Can you work these out from the model? Positions are in its coordinate system, mm. Round coordinates to 2 decimals unless told otherwise and drop trailing zeros. Write each loop counter-clockwise with the first axis right and the second up, starting at its lowest first coordinate (ties: lowest second). Pieces come first, ordered by that corner, then holes. Notation, with made-up numbers: M -1.5,-11.75 L 43.5,-11.75 A15 cw 43.5,9.25 Z; hole C 62.25,42 d5. An arc over 180 degrees is marked long. Answer as a JSON object with one key per item and string values. Group by question number.
1) Suppose I cut it at C-C, the plane z = -49.5. Write out the boundary of the cut face in (x, y).
2) Please list where these lines run through material, in increasing order: L1, parallel to Y at x = 0.65, z = -45; L2, parallel to Z at x = 0.2, y = -82; L3, parallel to Y at x = 0.6, z = -64. Write a range as [from, to].
3) Suppose I cut it at B-B, the plane y = -74. Write out the boundary of the cut face in (x, z).
4) Suppose I cut it at A-A, the plane x = 0.55. Write out the boundary of the cut face in (y, z), and give its area (3 significant figures).
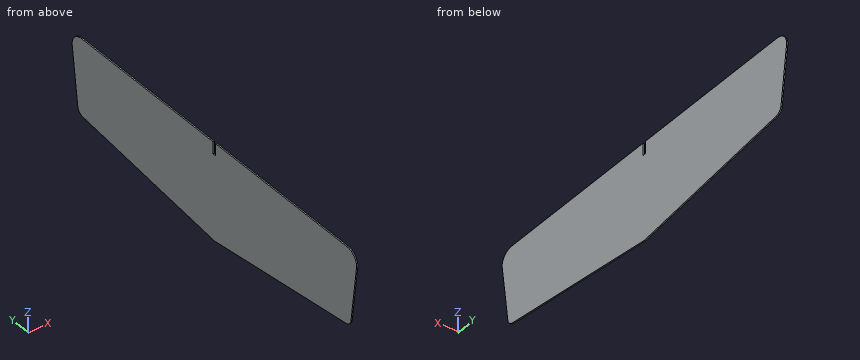
from build123d import *

# Parameters (mm, degrees)
F1_DEPTH = 1


# Not quite as in the source:
# - ends of sketch curves that miss each other by under 0.0002 mm in the source are joined


with BuildPart() as f1:
    # F0 (on Right) → F1 (new body)
    with BuildSketch(Plane.YZ):
        with BuildLine():
            Line((-17.710118, -7.110515), (-155.042295, -7.110515))
            ThreePointArc((-155.042295, -7.110515), (-162.539076635, -10.4924892282), (-164.9650738133, -18.3508619767))
            Line((-164.9650738133, -18.3508619767), (-159.139913, -64.952155))
            ThreePointArc((-159.139913, -64.952155), (-157.4251457547, -68.4543233257), (-153.91996093, -70.1629154318))
            Line((-153.91996093, -70.1629154318), (-16.370118, -87.110515))
            Line((-16.370118, -87.110515), (121.179726, -70.162916))
            ThreePointArc((121.179726, -70.162916), (124.6849107108, -68.4543233695), (126.3996771834, -64.9521550229))
            Line((126.3996771834, -64.9521550229), (132.224839, -18.350862))
            ThreePointArc((132.224839, -18.350862), (129.798841635, -10.4924892282), (122.30206, -7.110515))
            Line((122.30206, -7.110515), (-15.030118, -7.110515))
            Line((-15.030118, -7.110515), (-15.030118, -17.110515))
            Line((-15.030118, -17.110515), (-17.710118, -17.110515))
            Line((-17.710118, -17.110515), (-17.710118, -7.110515))
        make_face()
    extrude(amount=F1_DEPTH)


solid = f1.part
Results:
{
 "1": {"outline": "M 0,-161.07 L 1,-161.07 L 1,128.33 L 0,128.33 Z"},
 "2": {"L1": "[-161.63, 128.89]", "L2": "[-79.02, -7.11]", "L3": "[-159.26, 126.52]"},
 "3": {"outline": "M 0,-80.01 L 1,-80.01 L 1,-7.11 L 0,-7.11 Z"},
 "4": {"outline": "M -164.97,-18.35 L -159.14,-64.95 A6 ccw -153.92,-70.16 L -16.37,-87.11 L 121.18,-70.16 A6 ccw 126.4,-64.95 L 132.22,-18.35 A10 ccw 122.3,-7.11 L -15.03,-7.11 L -15.03,-17.11 L -17.71,-17.11 L -17.71,-7.11 L -155.04,-7.11 A10 ccw Z", "area": "20,700 mm^2"}
}
